```python
from build123d import *

# Parameters (mm, degrees)
BOSS_EXTRUDE2_DEPTH = 20
SKETCH3_R           = 7.5
CUT_EXTRUDE1_DEPTH  = 20
SKETCH4_R           = 20.021959316
BOSS_EXTRUDE3_DEPTH = 10
SKETCH5_R           = 15
CUT_EXTRUDE3_DEPTH  = 40


with BuildPart() as part:
    # Sketch1 → Boss-Extrude2 (new body)
    with BuildSketch(Plane.XY):
        with BuildLine():
            Line((111.70070007, 55.403547234), (-16.978506411, 55.403547234))
            ThreePointArc((-16.978506411, 55.403547234), (-25.627613379, 54.698491332), (-34.048339635, 52.601940713))
            Line((-34.048339635, 52.601940713), (-43.339871627, -25.020956816))
            ThreePointArc((-43.339871627, -25.020956816), (-2.457415402, -48.618782438), (38.425040824, -25.020956816))
            ThreePointArc((38.425040824, -25.020956816), (63.518057264, 16.418071125), (111.70070007, 21.446534413))
            ThreePointArc((111.70070007, 21.446534413), (128.67920648, 38.425040824), (111.70070007, 55.403547234))
        make_face()
    extrude(amount=BOSS_EXTRUDE2_DEPTH)

    # Sketch3 → Cut-Extrude1 (cut)
    with BuildSketch(Plane.XY.offset(20)):
        with Locations((-17.848919817, 38.425040824)):
            Circle(SKETCH3_R)
        with BuildLine():
            Line((54.895644648, 45.643601072), (111.70070007, 45.643601072))
            ThreePointArc((111.70070007, 45.643601072), (118.919260318, 38.425040824), (111.70070007, 31.206480576))
            Line((111.70070007, 31.206480576), (54.895644648, 31.206480576))
            ThreePointArc((54.895644648, 31.206480576), (47.6770844, 38.425040824), (54.895644648, 45.643601072))
        make_face()
    extrude(amount=-CUT_EXTRUDE1_DEPTH, mode=Mode.SUBTRACT)

    # Sketch4 → Boss-Extrude3 (add)
    with BuildSketch(Plane.XY.offset(20)):
        with Locations((0, -14.946583433)):
            Circle(SKETCH4_R)
    extrude(amount=BOSS_EXTRUDE3_DEPTH)

    # Sketch5 → Cut-Extrude3 (cut)
    with BuildSketch(Plane.XY.offset(30)):
        with Locations((0, -14.946583433)):
            Circle(SKETCH5_R)
    extrude(amount=-CUT_EXTRUDE3_DEPTH, mode=Mode.SUBTRACT)


solid = part.part
```
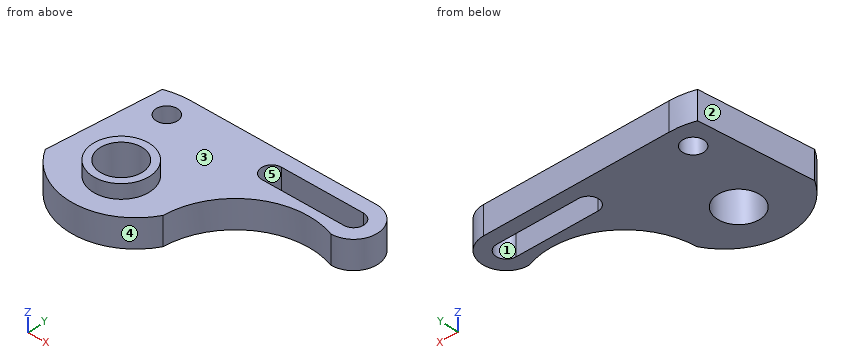
Design review of the part built by this model. Coordinates are the model's own, in mm. Face numbers are marked on the shaded views. A direction names the side the tool comes from. Round coordinates to 2 decimals unless told otherwise and drop trailing zeros. Order: outer loops, then holes, each group sorted by start corner. A loop starts at its lowest first (then second) coordinate and runs counter-clockwise, first axis right, second up. Notation, with made-up numbers: (-2, 66.25) - (14, 66.25) arc R31 cw to (14, 90.25) - close; hole circle Ø9 at (-6.75, 42). An arc over 180 degrees is marked (long way). One line per question, with ' | ' between items.
Item 1: Take a section at A-A, the plane x = 90. Write out the cut boundary in (y, z).
Checks:
outline: (24.82, 0) - (31.21, 0) - (31.21, 20) - (24.82, 20) - close; (45.64, 0) - (55.4, 0) - (55.4, 20) - (45.64, 20) - close
Item 2: Draft analysis for pull direction X (two halves, no side actions). For the marked faces 3, 4 and 5, state which applies: +X half, -X half, draft (parallel to the pull), parting line (faces both ways), or undercut.
Checks:
face 3: draft | face 4: parting line | face 5: undercut
Item 3: Wall thickness on line 1 (Y direction, x = 0, z = 21.25); line 2 (Z direction, x = 29.5, y = -34); line 3 (X direction, y = -10, z = 19.5): over which ranges is each line inside the solid? List them lowest first. Write a range as [from, to].
Checks:
line 1: [-34.97, -29.95], [0.05, 5.08] | line 2: [0, 20] | line 3: [-41.54, -14.16], [14.16, 41.87]
Item 4: Take a section at B-B, the plane y = 40.5. Write out the cut boundary in (x, z).
Checks:
outline: (-35.5, 0) - (-25.06, 0) - (-25.06, 20) - (-35.5, 20) - close; (-10.64, 0) - (47.98, 0) - (47.98, 20) - (-10.64, 20) - close; (118.61, 0) - (128.55, 0) - (128.55, 20) - (118.61, 20) - close
Item 5: Take a section at C-C, the plane z = 3. Write out the cut boundary in (x, y).
Checks:
outline: (-43.34, -25.02) arc R47.21 ccw to (38.43, -25.02) arc R54.43 cw to (111.7, 21.45) arc R16.98 ccw to (111.7, 55.4) - (-16.98, 55.4) arc R53.4 ccw to (-34.05, 52.6) - close; hole circle Ø15 at (-17.85, 38.43); hole circle Ø30 at (0, -14.95); hole (54.9, 31.21) - (111.7, 31.21) arc R7.22 ccw to (111.7, 45.64) - (54.9, 45.64) arc R7.22 ccw to start
Item 6: Machinability: for the marked faces 1 and 2, which of the approach directions +Z, -Z, +X, -X, +Y, -Y give a long, thin tool a straight path to every point of the face, cutting with its end or side? Answer none if there is none.
Checks:
face 1: +Z, -Z | face 2: +Z, -Z, -X, +Y
Item 7: For P1, Ø2, axis at y = 43, z = 15.5, coming from the -X side; P2, Ø5, axis at y = -19.5, z = 12, coming from the -X side; P3, Ø4, axis at x = 1.5, y = 23, coming from the +Z side; P4, Ø1.5, axis at x = 106.5, z = 21, coming from the +Y side, all flat-tipped, find the tip position at first contact; note any pin that passes through.
Checks:
P1: x = -35.32 | P2: x = -42.98 | P3: z = 20 | P4: through
Item 8: Take a section at D-D, the plane x = -1. Write out the cut boundary in (y, z).
Checks:
outline: (-48.6, 0) - (-29.91, 0) - (-29.91, 30) - (-34.94, 30) - (-34.94, 20) - (-48.6, 20) - close; (0.02, 0) - (55.4, 0) - (55.4, 20) - (5.05, 20) - (5.05, 30) - (0.02, 30) - close
